Work out the finished part from the listing and answer in its coordinate system (mm). A direction names the side the tool comes from. Give positions to 0.01 mm unless a question says otherwise; leave off trailing zeros. Loops run counter-clockwise (first coordinate to the right, second up) from the corner with the lowest first, then second, coordinate; pieces in that order, holes last. Notation, with made-up numbers: M 4,-21.5 L 43,-21.5 A14 cw 43,2.5 Z; hole C -16.5,33 d4. An arc over 180 degrees is marked long. Answer as a JSON object with one key per item and string values. Group by question number.
```python
from build123d import *

# Parameters (mm, degrees)
BOSS_EXTRUDE1_DEPTH = 15
BOSS_EXTRUDE2_DEPTH = 5
FILLET1_R           = 15
FILLET2_R           = 10
FILLET3_R           = 15


# Some blends are built 0.0001 mm under size
with BuildPart() as part:
    # Sketch1 → Boss-Extrude1 (new body)
    with BuildSketch(Plane.XY):
        Polygon((0, 0), (0, -50), (15, -50), (15, 0.565330323), (210.392182336, 35.018243889), (207.787459671, 49.790360184), (-28.566401052, 8.114797544), (-32.039364606, 27.810952604), (-41.887442136, 26.074470827), (-32, -30), (-32, -50), (-17, -50), (-17, 0), align=None)
    extrude(amount=BOSS_EXTRUDE1_DEPTH)

    # Sketch2 → Boss-Extrude2 (add)
    with BuildSketch(Plane.XY):
        Polygon((15, -50), (154.906481174, 25.23461773), (15, 0.565330323), align=None)
    extrude(amount=BOSS_EXTRUDE2_DEPTH)

    # Fillet1
    # the kernel refuses this fillet: 15 mm, written as the material it takes off along each edge
    with BuildSketch(Plane(origin=(-41.887442136, 26.074470827, -35.355339059), x_dir=(0.9848077530122078, 0.17364817766693189, 0), z_dir=(0, 0, 1))) as fillet1_piece_1:
        with BuildLine():
            CenterArc((15, -14.142135624), FILLET1_R, 109.471220634, 70.528779366)
            Line((0, -14.142135624), (-0.3, -14.142135624))
            Line((-0.3, -14.142135624), (-0.3, 0))
            Line((-0.3, 0), (0, 0.3))
            ThreePointArc((0, 0.3), (5, 0.3), (9.9, 0.282842712))
            Line((9.9, 0.282842712), (10, 0))
        make_face()
    extrude(amount=85.710678119, mode=Mode.SUBTRACT)

    # Fillet2
    fillet2_edges = [part.edges().sort_by_distance(p)[0] for p in [
        (-32, -50, 7.5),
    ]]
    fillet(fillet2_edges, radius=FILLET2_R)

    # Fillet3
    fillet3_edges = [part.edges().sort_by_distance(p)[0] for p in [
        (210.392182336, 35.018243889, 7.5),
    ]]
    fillet(fillet3_edges, radius=FILLET3_R - 0.0001)  # a hair under: the kernel refuses the full size


solid = part.part
```
Item 1: For a pull along X with two mould halves and no side action, classify faces 1 (the flat face through (15, -25, 10)), 2 (the flat face through (47, 8, 15)), 3 (the flat face through (0, -25, 7)), 4 (the flat face through (-17, -25, 7)) as pulls with the +X half, pulls with the -X half, needs draft (parallel to the pull), parting line crosses it, or undercut.
Item 2: A cutting plane is placed at C-C (x = 95.5). Determine the outline of the cut face in (y, z), and give its area (3 significant figures).
Item 3: Find the intervals of material crossed by probe 1 along X at (y, z) = (-40, 8.5); probe 2 along X at (y, z) = (-20.5, 10.25); probe 3 along Z at (x, y) = (34, -27), in increasing order. Write a range as [from, to].
Item 4: A tool of negligible diameter and unlimited length cuts with its end or side. For faces 5 (the flat face through (-32, -35, 7)), 6 (the flat face through (-9, 0, 7)), 7 (the flat face through (104.046, 16.266, 9.062)), 8 (the flat face through (91.265, 29.244, 7.395)), 9 (the flat face through (83.97, -12.91, 2.46)), from which of +Z, -Z, +X, -X, +Y, -Y can it reach the whole face along a straight path? Write none if from no direction.
Item 5: Given pin 1 Ø4.5 at (y, z) = (-34, 11) entering from +X; pin 2 Ø3 at (y, z) = (2.5, 3) entering from +X; pin 3 Ø2 at (x, z) = (69, 7) entering from +Y, each flat-ended and moving along its own axis, determine where each tip first touches the part or whether it passes through.
Item 6: A cutting plane is placed at D-D (y = -20.5). Determine the outline of the cut face in (x, z), and give its area (3 significant figures).
Item 7: A cutting plane is placed at A-A (y = -35). Determine the outline of the cut face in (x, z), and give its area (3 significant figures).
The answers:
{
 "1": {"face 1": "pulls with the +X half", "face 2": "needs draft", "face 3": "undercut", "face 4": "undercut"},
 "2": {"outline": "M -6.71,0 L 29.99,0 L 29.99,15 L 14.76,15 L 14.76,5 L -6.71,5 Z", "area": "336 mm^2"},
 "3": {"probe 1": "x = [-32, -17], [0, 15]", "probe 2": "x = [-33.68, -17], [0, 15]", "probe 3": "z = [0, 5]"},
 "4": {"face 5": "+Z, -Z, -X, -Y", "face 6": "+Z, -Z, -Y", "face 7": "+Z, +X, -Y", "face 8": "+Z, -Z, +Y", "face 9": "+Z, -Z, +X, -Y"},
 "5": {"pin 1": "stops at x = 15", "pin 2": "stops at x = 115.42", "pin 3": "stops at y = 25.49"},
 "6": {"outline": "M -33.68,0 L -17,0 L -17,15 L -33.68,15 Z; M 0,0 L 69.86,0 L 69.86,5 L 15,5 L 15,15 L 0,15 Z", "area": "749 mm^2"},
 "7": {"outline": "M -32,0 L -17,0 L -17,15 L -32,15 Z; M 0,0 L 42.89,0 L 42.89,5 L 15,5 L 15,15 L 0,15 Z", "area": "589 mm^2"}
}
